```python
from build123d import *

# Parameters (mm, degrees)
SKETCH3_R           = 4.25
SKETCH3_R_2         = 1.75
BOSS_EXTRUDE4_DEPTH = 3.675


with BuildPart() as part:
    # Sketch3 → Boss-Extrude4 (new, symmetric)
    with BuildSketch(Plane.XY):
        with BuildLine():
            ThreePointArc((-20.085093872, 75.379480002), (-37.522562339, 55.258676576), (-14.907803169, 41.205751446))
            Line((-14.907803169, 41.205751446), (35.902750732, 57.393327309))
            ThreePointArc((35.902750732, 57.393327309), (42.069224422, 67.316764326), (33.240144084, 74.968387709))
            Line((33.240144084, 74.968387709), (-20.085093872, 75.379480002))
        make_face()
        with Locations((-20.22, 57.88)):
            Circle(SKETCH3_R, mode=Mode.SUBTRACT)
        with Locations((33.17076379, 65.968655136)):
            Circle(SKETCH3_R_2, mode=Mode.SUBTRACT)
    extrude(amount=BOSS_EXTRUDE4_DEPTH, both=True)


solid = part.part
```
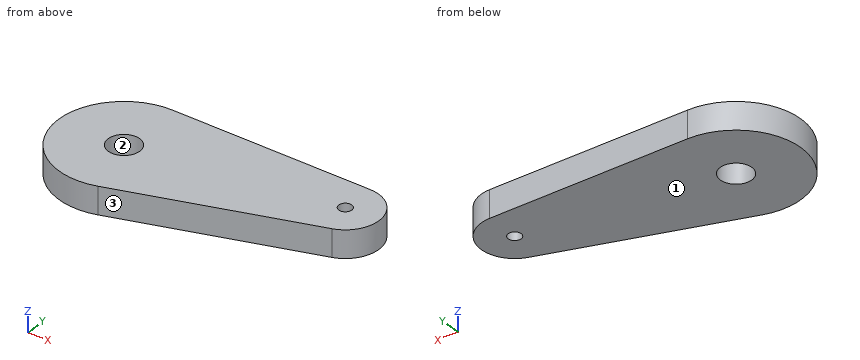
Source: CAD feature listing. Evaluate the final solid. Frame: model axes, mm. Face numbers are marked on the shaded views. Give positions to 0.01 mm unless a question says otherwise; leave off trailing zeros. Order: outer loops, then holes, each group sorted by start corner. A loop starts at its lowest first (then second) coordinate and runs counter-clockwise, first axis right, second up. Notation, with made-up numbers: (76, -23.75) -> (81, -23.75) arc R37 ccw to (81, 13.25) -> close; hole circle Ø8 at (23.25, -14.75). An arc over 180 degrees is marked (long way). Use a Markdown table: item, result.
Q1. Section C-C (z = 0.5). Return the cut outline in (x, y).
A:
| item | result |
|---|---|
| outline | (-20.09, 75.38) arc R17.5 ccw (long way) to (-14.91, 41.21) -> (35.9, 57.39) arc R9 ccw to (33.24, 74.97) -> close; hole circle Ø8.5 at (-20.22, 57.88); hole circle Ø3.5 at (33.17, 65.97) |
Q2. Section B-B (x = -21.5). Return the cut outline in (y, z) (3 decimals), and give its area (3 significant figures).
A:
| item | result |
|---|---|
| outline | (40.427, -3.675) -> (53.827, -3.675) -> (53.827, 3.675) -> (40.427, 3.675) -> close; (61.933, -3.675) -> (75.333, -3.675) -> (75.333, 3.675) -> (61.933, 3.675) -> close |
| area | 197 mm^2 |
Q3. Pull-direction query (X, two-part tool) for the marked faces 1, 2 and 3; classes: +X half, -X half, draft (parallel to the pull), parting line (faces both ways), or undercut.
A:
| item | result |
|---|---|
| face 1 | draft |
| face 2 | undercut |
| face 3 | +X half |
Q4. Material intervals for line 1 (Y direction, x = -20.22, z = 0.75); line 2 (X direction, y = 61, z = 0.25); line 3 (X direction, y = 60, z = -2.5), sorted ascending. Write a range as [from, to].
A:
| item | result |
|---|---|
| line 1 | [40.38, 53.63], [62.13, 75.38] |
| line 2 | [-37.44, -23.11], [-17.33, 40.67] |
| line 3 | [-37.59, -23.9], [-16.54, 39.91] |
Q5. Section D-D (y = 68.5). Return the cut outline in (x, z) (3 decimals).
A:
| item | result |
|---|---|
| outline | (-34.129, -3.675) -> (41.807, -3.675) -> (41.807, 3.675) -> (-34.129, 3.675) -> close |
Q6. Section A-A (y = 56.5). Return the cut outline in (x, z) (1 decimal).
A:
| item | result |
|---|---|
| outline | (-37.7, -3.7) -> (-24.2, -3.7) -> (-24.2, 3.7) -> (-37.7, 3.7) -> close; (-16.2, -3.7) -> (33.1, -3.7) -> (33.1, 3.7) -> (-16.2, 3.7) -> close |
Q7. First-contact query: P1, Ø1.5, axis at x = -11.5, z = -2.5, coming from the +Y side; P2, Ø11, axis at x = -20.22, y = 57.88, coming from the +Z side (3 decimals); P3, Ø1.5, axis at x = -18, z = 1.5, coming from the +Y side; P4, Ø4, axis at x = -22.5, z = 2, coming from the -Y side. Flat tips, straight axial feed; report the tip coordinate or a pass-through.
A:
| item | result |
|---|---|
| P1 | y = 75.32 |
| P2 | z = 3.675 |
| P3 | y = 75.37 |
| P4 | y = 40.38 |
